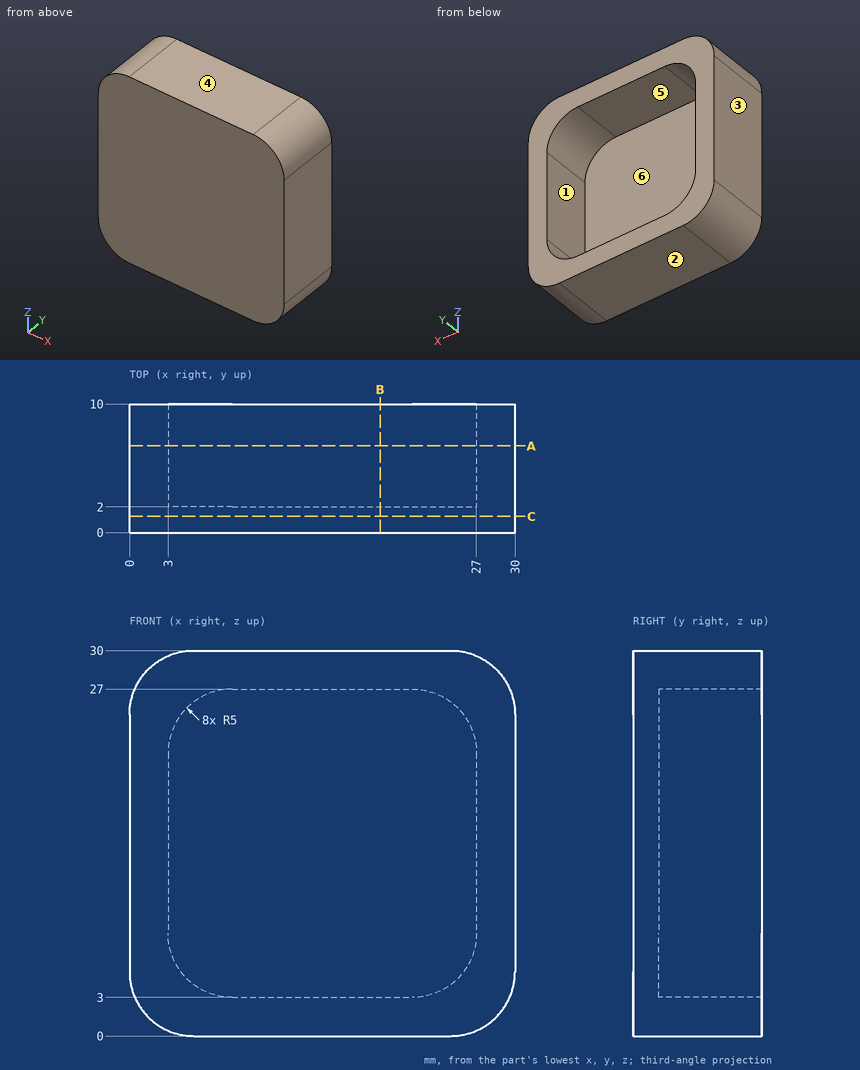
Verification items for this drawing (mm, ordinates from the low corner). A direction names the side the tool comes from. Give positions to 0.01 mm unless a question says otherwise; leave off trailing zeros. Write each loop counter-clockwise with the first axis right and the second up, starting at its lowest first coordinate (ties: lowest second). Pieces come first, ordered by that corner, then holes. Notation, with made-up numbers: (20.25, 26.25) - (42.25, 26.25) arc R19 cw to (42.25, 30.25) - close; hole circle Ø6 at (-23.5, 4). An arc over 180 degrees is marked (long way). Answer as CSV lines item,"result". Start each with the question number.
1. Draft check along Z on the marked faces 3, 4, 5 and 6. Enter one of: pulls with the +Z half, pulls with the -Z half, needs draft (parallel to the pull), parting line crosses it, or undercut.
2. Sectioned sample at B-B (x = 19.5). Record the boundary of the cut face in (y, z).
3. Sectioned sample at C-C (y = 1.25). Record the boundary of the cut face in (x, z), then the cut area to 3 significant figures.
4. Set-up check for the marked faces 1 and 2: record each of +Z, -Z, +X, -X, +Y, -Y from which the full face is reachable in a straight line by a thin tool's end or side.
5. Depth check by flat-ended pin: pin 1 (4 mm diameter, centred on y = 3, z = 6.5, fed in from -X); pin 2 (7 mm diameter, centred on x = 21, z = 16, fed in from +Y). Enter the tip coordinate at first touch or a pass-through.
6. Thickness scan on line 1 (X direction, y = 4.5, z = 19.75); line 2 (Y direction, x = 15.25, z = 16.75). Record the ranges inside material, lowest first.
7. Sectioned sample at A-A (y = 6.75). Record the boundary of the cut face in (x, z).
Derived:
1,face 3,"needs draft"
1,face 4,"pulls with the +Z half"
1,face 5,"undercut"
1,face 6,"undercut"
2,outline,"(0, 0) - (10, 0) - (10, 3) - (2, 3) - (2, 27) - (10, 27) - (10, 30) - (0, 30) - close"
3,outline,"(0, 5) arc R5 ccw to (5, 0) - (25, 0) arc R5 ccw to (30, 5) - (30, 25) arc R5 ccw to (25, 30) - (5, 30) arc R5 ccw to (0, 25) - close"
3,area,"879 mm²"
4,face 1,"+Y"
4,face 2,"-Z, +X, -X, +Y, -Y"
5,pin 1,"x = 0"
5,pin 2,"y = 2"
6,line 1,"0 to 3, 27 to 30"
6,line 2,"0 to 2"
7,outline,"(0, 5) arc R5 ccw to (5, 0) - (25, 0) arc R5 ccw to (30, 5) - (30, 25) arc R5 ccw to (25, 30) - (5, 30) arc R5 ccw to (0, 25) - close; hole (3, 8) arc R5 ccw to (8, 3) - (22, 3) arc R5 ccw to (27, 8) - (27, 22) arc R5 ccw to (22, 27) - (8, 27) arc R5 ccw to (3, 22) - close"
